```python
from build123d import *

# Parameters (mm, degrees)
SKETCH1_R           = 24
SKETCH1_R_2         = 22
BOSS_EXTRUDE1_DEPTH = 5
BOSS_EXTRUDE2_DEPTH = 2
SKETCH3_R           = 2
BOSS_EXTRUDE3_DEPTH = 2


with BuildPart() as part:
    # Sketch1 → Boss-Extrude1 (new body)
    with BuildSketch(Plane(origin=(0, 0, 0), x_dir=(1, 0, 0), z_dir=(0, 1, 0))):
        with Locations(Location((0, 0, 0), (0, 0, 270))):
            Circle(SKETCH1_R)
        with Locations(Location((0, 0, 0), (0, 0, 270))):
            Circle(SKETCH1_R_2, mode=Mode.SUBTRACT)
    extrude(amount=BOSS_EXTRUDE1_DEPTH)

    # Sketch2 → Boss-Extrude2 (add)
    with BuildSketch(Plane.XZ):
        with BuildLine():
            Line((-18.126828112, 12.833489636), (-18.126828112, 15.729529636))
            ThreePointArc((-18.126828112, 15.729529636), (-24, 0), (-18.126828112, -15.729529636))
            Line((-18.126828112, -15.729529636), (-18.126828112, -12.833489636))
            ThreePointArc((-18.126828112, -12.833489636), (-22.209915661, 0), (-18.126828112, 12.833489636))
        make_face()
        with BuildLine():
            Line((-18.126828112, -12.466679694), (-18.126828112, 12.466679694))
            ThreePointArc((-18.126828112, 12.466679694), (-22, 0), (-18.126828112, -12.466679694))
        make_face()
        with BuildLine():
            ThreePointArc((-10.126828112, 19.530677213), (-12.199845938, 18.307478229), (-14.126828112, 16.865133485))
            Line((-14.126828112, 16.865133485), (-14.126828112, -16.865133485))
            ThreePointArc((-14.126828112, -16.865133485), (-12.199845938, -18.307478229), (-10.126828112, -19.530677213))
            Line((-10.126828112, -19.530677213), (-10.126828112, 19.530677213))
        make_face()
        with BuildLine():
            ThreePointArc((-2.126828112, 21.896954176), (-4.14462307, 21.606066269), (-6.126828112, 21.12964688))
            Line((-6.126828112, 21.12964688), (-6.126828112, -21.12964688))
            ThreePointArc((-6.126828112, -21.12964688), (-4.14462307, -21.606066269), (-2.126828112, -21.896954176))
            Line((-2.126828112, -21.896954176), (-2.126828112, 21.896954176))
        make_face()
        with BuildLine():
            ThreePointArc((5.873171888, 21.201553056), (3.889799677, 21.653393694), (1.873171888, 21.920110106))
            Line((1.873171888, 21.920110106), (1.873171888, -21.920110106))
            ThreePointArc((1.873171888, -21.920110106), (3.889799677, -21.653393694), (5.873171888, -21.201553056))
            Line((5.873171888, -21.201553056), (5.873171888, 21.201553056))
        make_face()
        with BuildLine():
            ThreePointArc((13.873171888, 17.074399017), (11.943353973, 18.475830045), (9.873171888, 19.66012403))
            Line((9.873171888, 19.66012403), (9.873171888, -19.66012403))
            ThreePointArc((9.873171888, -19.66012403), (11.943353973, -18.475830045), (13.873171888, -17.074399017))
            Line((13.873171888, -17.074399017), (13.873171888, 17.074399017))
        make_face()
        with BuildLine():
            ThreePointArc((22, 0), (20.94289595, 6.737589275), (17.873171888, 12.82769374))
            Line((17.873171888, 12.82769374), (17.873171888, -12.82769374))
            ThreePointArc((17.873171888, -12.82769374), (20.94289595, -6.737589275), (22, 0))
        make_face()
    extrude(amount=-BOSS_EXTRUDE2_DEPTH)

    # Sketch3 → Boss-Extrude3 (add)
    # profile 1 of 2: a face of its own
    with BuildSketch(Plane(origin=(0, 5, 0), x_dir=(1, 0, 0), z_dir=(0, 1, 0))):
        with BuildLine():
            Line((-28, 4), (-22.866655367, 4))
            Line((-22.866655367, 4), (-22.866655367, -4))
            Line((-22.866655367, -4), (-28, -4))
            ThreePointArc((-28, -4), (-32, 0), (-28, 4))
        make_face()
        with Locations(Location((-28, 0, 0), (0, 0, 270))):
            Circle(SKETCH3_R, mode=Mode.SUBTRACT)
    # profile 2 of 2: a face of its own
    with BuildSketch(Plane(origin=(0, 5, 0), x_dir=(1, 0, 0), z_dir=(0, 1, 0))):
        with BuildLine():
            Line((-4, 22.866655367), (-4, 28))
            ThreePointArc((-4, 28), (0, 32), (4, 28))
            Line((4, 28), (4, 22.866655367))
            Line((4, 22.866655367), (-4, 22.866655367))
        make_face()
        with Locations(Location((0, 28, 0), (0, 0, 270))):
            Circle(SKETCH3_R, mode=Mode.SUBTRACT)
    extrude(amount=-BOSS_EXTRUDE3_DEPTH)


solid = part.part
```
Verification items for the finished model (mm, model axes). A direction names the side the tool comes from. Round coordinates to 2 decimals unless told otherwise and drop trailing zeros. Write each loop counter-clockwise with the first axis right and the second up, starting at its lowest first coordinate (ties: lowest second). Pieces come first, ordered by that corner, then holes.
1. Draft check along Y on faces 6 (the flat face through (12, 2, 0)), 7 (the flat face through (-5, 0, 0)), 8 (the cylindrical face through (-32, 4, 0)). Enter one of: +Y half, -Y half, draft (parallel to the pull), parting line (faces both ways), or undercut.
2. Section check A-A on x = 0. Enter the section's corners in (y, z).
3. Gauge pin test, flat ends, axial feed: P1, Ø1.6, axis at y = 1, z = 3, coming from the -X side; P2, Ø1, axis at y = 3, z = 10, coming from the -X side; P3, Ø4, axis at x = -28, z = 1.5, coming from the -Y side. Record the tip position at first contact, or that the pin passes through.
4. Section check D-D on z = -10.5. Enter the section's corners in (x, y), plus the area to 3 significant figures.
5. Section check B-B on z = 0. State how many separate pieces and enclosed holes the cut face has, plus the area to 3 significant figures.
6. Section check C-C on y = 4.25. Enter the section's corners in (x, z).
7. Access from +Z, -Z, +X, -X, +Y, -Y to the whole of each face (thin tool, end or side, straight path). Record for faces 1 (the flat face through (-26, 4, -4)), 2 (the flat face through (-26, 4, 4)), 3 (the flat face through (-12, 5, -19)), 4 (the flat face through (-20, 2, 0)), 5 (the flat face through (-14.127, 1, 0)).
8. Scan lines: L1, parallel to X at y = 3.65, z = 0; L2, parallel to Z at x = 0, y = 2.9; L3, parallel to X at y = 2.3, z = -0.5. Record each from-to range of solid material in increasing order.
Answer:
1. face 6: +Y half
1. face 7: -Y half
1. face 8: draft
2. outline: (0, -24) - (3, -24) - (3, -26) - (5, -26) - (5, -22) - (0, -22) - close; (0, 22) - (5, 22) - (5, 24) - (0, 24) - close; (3, -32) - (5, -32) - (5, -30) - (3, -30) - close
3. P1: stops at x = -23.9
3. P2: stops at x = -22.04
3. P3: stops at y = 3
4. outline: (-21.58, 0) - (-18.13, 0) - (-18.13, 2) - (-19.33, 2) - (-19.33, 5) - (-21.58, 5) - close; (-14.13, 0) - (-10.13, 0) - (-10.13, 2) - (-14.13, 2) - close; (-6.13, 0) - (-2.13, 0) - (-2.13, 2) - (-6.13, 2) - close; (1.87, 0) - (5.87, 0) - (5.87, 2) - (1.87, 2) - close; (9.87, 0) - (13.87, 0) - (13.87, 2) - (9.87, 2) - close; (17.87, 0) - (21.58, 0) - (21.58, 5) - (19.33, 5) - (19.33, 2) - (17.87, 2) - close
4. area: 59.8 mm2
5. separate pieces: 7
5. enclosed holes: 0
5. area: 76.0 mm2
6. outline: (-28, -4) - (-23.66, -4) arc R24 ccw to (-4, -23.66) - (-4, -28) arc R4 ccw to (4, -28) - (4, -23.66) arc R24 ccw (long way) to (-23.66, 4) - (-28, 4) arc R4 ccw to start; hole circle Ø4 at (-28, 0); hole circle Ø44 at (0, 0); hole circle Ø4 at (0, -28)
7. face 1: -Z, -X, +Y, -Y
7. face 2: +Z, -X, +Y, -Y
7. face 3: +Z, -Z, +X, -X, +Y
7. face 4: +Y
7. face 5: +Y, -Y
8. L1: x = -32 to -30, -26 to -22, 22 to 24
8. L2: z = -24 to -22, 22 to 24
8. L3: x = -23.99 to -21.99, 21.99 to 23.99
